Part model, mm, in its own coordinate system. A direction names the side the tool comes from. Give positions to 0.01 mm unless a question says otherwise; leave off trailing zeros. Write each loop counter-clockwise with the first axis right and the second up, starting at its lowest first coordinate (ties: lowest second). Pieces come first, ordered by that corner, then holes. Notation, with made-up numbers: M 42.5,49 L 52.5,49 A18 ccw 52.5,72 Z; hole C -38.75,-39 d7. An arc over 180 degrees is marked long. Use CSV: the item, a comma, the result in double quotes. Start each with the question number.
1. Drop flat-ended pins along their axis: pin 1 Ø3.5 at (x, z) = (-26.67, 34.925) entering from -Y; pin 2 Ø9 at (x, z) = (0.5, 12) entering from +Y. Give the stop position or say it passes through.
2. Band-saw the part on B-B, the plane z = 15.24. List the corners of the cut face in (x, y), then the cut area to 3 significant figures.
3. Band-saw the part on A-A, the plane x = -26.67. List the corners of the cut face in (y, z), then the cut area to 3 significant figures.
4. Mould opens along X. For faces 1 (the face through (31.75, -10, 20)), 2 (the face through (-31.75, -10, 20)), 3 (the face through (0, -10, 39.624)), 4 (the face through (25, -9.906, 15)) say: pulls with the +X half, pulls with the -X half, needs draft (parallel to the pull), parting line crosses it, or undercut.
5. Band-saw the part on D-D, the plane x = 0. List the corners of the cut face in (y, z).
6. Drill centre lines: line 1 along X through (y, z) = (-9.1, 15.24); line 2 along X through (y, z) = (-9.25, 33.5); line 3 along Z through (x, y) = (-26.67, -11.5). Where is each one in solid material? Low to high. Write a range as from..to.
7. Band-saw the part on C-C, the plane y = -8. Count the separate pieces of the cut face and the enclosed holes in it, then the cut area to 3 significant figures.
8. 3-axis set-ups, long thin cutter, end or side, ignore diameter. For faces 5 (the face through (-21.617, -8.153, 15.653)), 6 (the face through (-8, -6.35, 24)): which of +Z, -Z, +X, -X, +Y, -Y reach the whole face in a straight line?
from build123d import *

# Parameters (mm, degrees)
SKETCH1_W           = 63.5
SKETCH1_H           = 25.4
BOSS_EXTRUDE1_DEPTH = 38.1
SKETCH2_R           = 3.175
CUT_EXTRUDE1_DEPTH  = 12.7
SKETCH2_3_R         = 8.763
CUT_EXTRUDE2_DEPTH  = 4.826
CUT_EXTRUDE3_START  = -20.574
SKETCH3_R           = 6.35
CUT_EXTRUDE3_DEPTH  = 20.574
SKETCH4_R           = 10.795
CUT_EXTRUDE4_DEPTH  = 19.05
SKETCH5_R           = 1.5875
CUT_EXTRUDE5_DEPTH  = 50.8
SKETCH6_W           = 63.5
SKETCH6_H           = 1.27
CUT_EXTRUDE6_DEPTH  = 38.1
SKETCH7_W           = 63.5
SKETCH7_H           = 24.13
BOSS_EXTRUDE2_DEPTH = 1.524
SKETCH8_W           = 95.143419866
SKETCH8_H           = 69.172862942
CUT_EXTRUDE7_DEPTH  = 55.231230633
SKETCH9_W           = 63.5
SKETCH9_H           = 39.624
SKETCH9_R           = 1.5875
SKETCH9_R_2         = 3.175
SKETCH9_R_3         = 8.763
BOSS_EXTRUDE3_DEPTH = 2.54
SKETCH10_R          = 8.763
SKETCH10_R_2        = 6.35
CUT_EXTRUDE9_DEPTH  = 52.343824127
SKETCH11_R          = 8.763
SKETCH11_R_2        = 3.175
BOSS_EXTRUDE5_DEPTH = 4.064


with BuildPart() as part:
    # Sketch1 → Boss-Extrude1 (new body)
    with BuildSketch(Plane.XY):
        Rectangle(SKETCH1_W, SKETCH1_H)
    extrude(amount=BOSS_EXTRUDE1_DEPTH)

    # Sketch2 → Cut-Extrude1 (cut)
    with BuildSketch(Plane.XZ.offset(12.7)):
        with Locations(Location((-24.765, 15.24, 0), (0, 0, 270))):
            Circle(SKETCH2_R)
        with Locations(Location((24.765, 15.24, 0), (0, 0, 270))):
            Circle(SKETCH2_R)
    extrude(amount=-CUT_EXTRUDE1_DEPTH, mode=Mode.SUBTRACT)

    # Sketch2<3> → Cut-Extrude2 (cut)
    with BuildSketch(Plane.XZ.offset(12.7)):
        with Locations(Location((0, 15.24, 0), (0, 0, 270))):
            Circle(SKETCH2_3_R)
    extrude(amount=-CUT_EXTRUDE2_DEPTH, mode=Mode.SUBTRACT)

    # Sketch3 → Cut-Extrude3 (cut)
    with BuildSketch(Plane.XZ.offset(7.874).offset(CUT_EXTRUDE3_START)):
        with Locations(Location((0, 15.24, 0), (0, 0, 270))):
            Circle(SKETCH3_R)
    extrude(amount=CUT_EXTRUDE3_DEPTH, mode=Mode.SUBTRACT)

    # Sketch4 → Cut-Extrude4 (cut)
    with BuildSketch(Plane(origin=(0, 12.7, 0), x_dir=(1, 0, 0), z_dir=(0, 1, 0))):
        with Locations(Location((0, -15.24, 0), (0, 0, 270))):
            Circle(SKETCH4_R)
    extrude(amount=-CUT_EXTRUDE4_DEPTH, mode=Mode.SUBTRACT)

    # Sketch5 → Cut-Extrude5 (cut)
    with BuildSketch(Plane(origin=(0, 12.7, 0), x_dir=(1, 0, 0), z_dir=(0, 1, 0))):
        with Locations(Location((-26.67, -34.925, 0), (0, 0, 270))):
            Circle(SKETCH5_R)
        with Locations(Location((0, -34.925, 0), (0, 0, 270))):
            Circle(SKETCH5_R)
        with Locations(Location((26.67, -34.925, 0), (0, 0, 270))):
            Circle(SKETCH5_R)
    extrude(amount=-CUT_EXTRUDE5_DEPTH, mode=Mode.SUBTRACT)

    # Sketch6 → Cut-Extrude6 (cut)
    with BuildSketch(Plane.XY.offset(38.1)):
        with Locations((0, -12.065)):
            Rectangle(SKETCH6_W, SKETCH6_H)
    extrude(amount=-CUT_EXTRUDE6_DEPTH, mode=Mode.SUBTRACT)

    # Sketch7 → Boss-Extrude2 (add)
    with BuildSketch(Plane.XY.offset(38.1)):
        with Locations((0, 0.635)):
            Rectangle(SKETCH7_W, SKETCH7_H)
    extrude(amount=BOSS_EXTRUDE2_DEPTH)

    # Sketch8 → Cut-Extrude7 (cut, through all)
    with BuildSketch(Plane(origin=(0, -6.35, 0), x_dir=(1, 0, 0), z_dir=(0, 1, 0))):
        with Locations((5.084942731, -21.829519101)):
            Rectangle(SKETCH8_W, SKETCH8_H)
    extrude(amount=CUT_EXTRUDE7_DEPTH, mode=Mode.SUBTRACT)

    # Sketch9 → Boss-Extrude3 (add)
    with BuildSketch(Plane.XZ.offset(11.43)):
        with Locations((0, 19.812)):
            Rectangle(SKETCH9_W, SKETCH9_H)
        with Locations(Location((26.67, 34.925, 0), (0, 0, 90))):
            Circle(SKETCH9_R, mode=Mode.SUBTRACT)
        with Locations(Location((0, 34.925, 0), (0, 0, 90))):
            Circle(SKETCH9_R, mode=Mode.SUBTRACT)
        with Locations(Location((-26.67, 34.925, 0), (0, 0, 90))):
            Circle(SKETCH9_R, mode=Mode.SUBTRACT)
        with Locations(Location((-24.765, 15.24, 0), (0, 0, 270))):
            Circle(SKETCH9_R_2, mode=Mode.SUBTRACT)
        with Locations(Location((0, 15.24, 0), (0, 0, 270))):
            Circle(SKETCH9_R_3, mode=Mode.SUBTRACT)
        with Locations(Location((24.765, 15.24, 0), (0, 0, 270))):
            Circle(SKETCH9_R_2, mode=Mode.SUBTRACT)
    extrude(amount=BOSS_EXTRUDE3_DEPTH)

    # Sketch10 → Cut-Extrude9 (cut, through all)
    with BuildSketch(Plane.XZ.offset(13.97)):
        with Locations(Location((0, 15.24, 0), (0, 0, 270))):
            Circle(SKETCH10_R)
        with Locations((0, 15.24)):
            Circle(SKETCH10_R_2, mode=Mode.SUBTRACT)
    extrude(amount=-CUT_EXTRUDE9_DEPTH, mode=Mode.SUBTRACT)

    # Sketch11 → Boss-Extrude5 (add)
    with BuildSketch(Plane.XZ.offset(13.97)):
        with Locations(Location((0, 15.24, 0), (0, 0, 270))):
            Circle(SKETCH11_R)
        with Locations(Location((24.765, 15.24, 0), (0, 0, 270))):
            Circle(SKETCH11_R_2)
        with Locations(Location((-24.765, 15.24, 0), (0, 0, 270))):
            Circle(SKETCH11_R_2)
    extrude(amount=-BOSS_EXTRUDE5_DEPTH)


solid = part.part
Output:
1,pin 1,"stops at y = -13.97"
1,pin 2,"stops at y = -9.91"
2,outline,"M -31.75,-13.97 L 31.75,-13.97 L 31.75,-6.35 L 27.94,-6.35 L 27.94,-9.91 L 21.59,-9.91 L 21.59,-6.35 L 8.76,-6.35 L 8.76,-9.91 L -8.76,-9.91 L -8.76,-6.35 L -21.59,-6.35 L -21.59,-9.91 L -27.94,-9.91 L -27.94,-6.35 L -31.75,-6.35 Z"
2,area,"376 mm²"
3,outline,"M -13.97,0 L -6.35,0 L -6.35,12.7 L -9.91,12.7 L -9.91,17.78 L -6.35,17.78 L -6.35,33.34 L -13.97,33.34 Z; M -13.97,36.51 L -6.35,36.51 L -6.35,39.62 L -13.97,39.62 Z"
3,area,"260 mm²"
4,face 1,"pulls with the +X half"
4,face 2,"pulls with the -X half"
4,face 3,"needs draft"
4,face 4,"undercut"
5,outline,"M -13.97,0 L -6.35,0 L -6.35,6.48 L -9.91,6.48 L -9.91,24 L -6.35,24 L -6.35,33.34 L -13.97,33.34 Z; M -13.97,36.51 L -6.35,36.51 L -6.35,39.62 L -13.97,39.62 Z"
6,line 1,"x = -31.75..-27.94, -21.59..-8.76, 8.76..21.59, 27.94..31.75"
6,line 2,"x = -31.75..-27.37, -25.97..-0.7, 0.7..25.97, 27.37..31.75"
6,line 3,"z = 0..33.34, 36.51..39.62"
7,separate pieces,"1"
7,enclosed holes,"6"
7,area,"2,190 mm²"
8,face 5,"+Y"
8,face 6,"+Z, -Z, +X, -X, +Y"
